Check sheet for the modelled part. Datum: model origin and axes. Units: mm. A direction names the side the tool comes from. Coordinates: 2 decimals unless noted, no trailing zeros. Loops run counter-clockwise (first coordinate to the right, second up) from the corner with the lowest first, then second, coordinate; pieces in that order, holes last. Notation, with made-up numbers: M -31.75,87 L 4.25,87 A18 ccw 4.25,92 Z; hole C -36.75,-27.75 d2. An arc over 180 degrees is marked long. Answer in a Markdown table with one row per item. Add a question column.
```python
from build123d import *

# Parameters (mm, degrees)
F0_W      = 50.8
F0_H      = 50.8
F1_DEPTH  = 4.13
F3_W      = 45.72
F3_H      = 45.72
F4_DEPTH  = 3.77
F5_W      = 8
F5_H      = 23.114
F6_DEPTH  = 3.2
F7_R      = 1.715
F8_DEPTH  = 25.4
F9_SIZE   = 1.27
F10_R     = 1.694213851
F11_DEPTH = 25.4


# Not quite as in the source:
# - a feature names something its author has since deleted; it is built from what else it names


with BuildPart() as f1:
    # F0 (on Top) → F1 (new body)
    with BuildSketch(Plane.XY):
        with Locations((13.0843408406, 14.7212249442)):
            Rectangle(F0_W, F0_H)
    extrude(amount=F1_DEPTH)

    # F3 (on face) → F4 (join)
    with BuildSketch(Plane.XY.offset(4.13)):
        with Locations((13.0843408406, 14.7212249442)):
            Rectangle(F3_W, F3_H)
    extrude(amount=F4_DEPTH)

    # F5 (on face) → F6 (cut)
    with BuildSketch(Plane.XY.offset(7.9)):
        with Locations((4.2001288666, 14.5942249442)):
            Rectangle(F5_W, F5_H)
        with Locations((13.0901288666, 14.5942249442)):
            Rectangle(F5_W, F5_H)
        with Locations((21.9801288666, 14.5942249442)):
            Rectangle(F5_W, F5_H)
        with Locations((30.8701288666, 14.5942249442)):
            Rectangle(F5_W, F5_H)
        with Locations((-4.6898711334, 14.5942249442)):
            Rectangle(F5_W, F5_H)
    extrude(amount=-F6_DEPTH, mode=Mode.SUBTRACT)

    # F7 (on face) → F8 (cut)
    with BuildSketch(Plane.XY.offset(4.7)):
        with Locations((-4.6898711334, 7.9362249442)):
            Circle(F7_R)
    extrude(amount=-F8_DEPTH, mode=Mode.SUBTRACT)

    # F9
    f9_edges = [f1.edges().sort_by_distance(p)[0] for p in [
        (13.084341, -10.678775, 0),
        (13.084341, 40.121225, 0),
        (-12.315659, 14.721225, 0),
        (38.484341, 14.721225, 0),
    ]]
    chamfer(f9_edges, length=F9_SIZE)

    # F10 (on face) → F11 (cut)
    with BuildSketch(Plane.XY.offset(4.7)):
        with Locations((4.1879288666, 7.9312249442)):
            Circle(F10_R)
        with Locations((13.0779288666, 7.9312249442)):
            Circle(F10_R)
        with Locations((21.9679288666, 7.9312249442)):
            Circle(F10_R)
        with Locations((30.8579288666, 7.9394249442)):
            Circle(F10_R)
    extrude(amount=-F11_DEPTH, mode=Mode.SUBTRACT)


solid = f1.part
```
Q1. Access from +Z, -Z, +X, -X, +Y, -Y to the whole of each face (thin tool, end or side, straight path). Record for faces 1 (the face through (20.275, 8.006, 2.383)), 2 (the face through (-9.776, 14, 6)), 3 (the face through (31, 15, 4.7)).
Q2. Cross-section at B-B (x = 22). Record the cut outline in (y, z).
Q3. Cross-section at D-D (x = 16.5). Record the cut outline in (y, z).
Q4. Thickness scan on L1, parallel to X at y = 14.5, z = 7.25; L2, parallel to Y at x = 18.5, z = 7; L3, parallel to Z at x = -8.5, y = 7. Record the ranges inside material, lowest first.
Q5. Cross-section at A-A (z = 6.75). Record the cut outline in (x, y), plus the area to 3 significant figures.
Q6. Go/stop test with flat-tipped pins: pin 1 (1 mm diameter, centred on x = 30, z = 6.5, fed in from +Y); pin 2 (1.5 mm diameter, centred on y = 22, z = 1, fed in from +X); pin 3 (1.6 mm diameter, centred on y = 18.5, z = 6.5, fed in from +X); pin 4 (1.9 mm diameter, centred on y = 13.5, z = 5.5, fed in from -X). Record where each tip stops, or that it passes through.
Q7. Mould release check, pull along X, two halves, no side actions. Record for faces 4 (the face through (13, -10.679, 3)), 5 (the face through (-12.316, 14, 3)), 6 (the face through (8.2, 14, 6)): released by +X, released by -X, zero draft, split by the parting line, or undercut.
Q8. Cross-section at C-C (y = 29). Record the cut outline in (x, z).
Answer key:
| question | item | result |
|---|---|---|
| 1 | face 1 | +Z, -Z |
| 1 | face 2 | +Z, -X, +Y, -Y |
| 1 | face 3 | +Z |
| 2 | outline | M -10.68,1.27 L -9.41,0 L 6.24,0 L 6.24,4.7 L 3.04,4.7 L 3.04,7.9 L -8.14,7.9 L -8.14,4.13 L -10.68,4.13 Z; M 9.63,0 L 38.85,0 L 40.12,1.27 L 40.12,4.13 L 37.58,4.13 L 37.58,7.9 L 26.15,7.9 L 26.15,4.7 L 9.63,4.7 Z |
| 3 | outline | M -10.68,1.27 L -9.41,0 L 38.85,0 L 40.12,1.27 L 40.12,4.13 L 37.58,4.13 L 37.58,7.9 L 26.15,7.9 L 26.15,4.7 L 3.04,4.7 L 3.04,7.9 L -8.14,7.9 L -8.14,4.13 L -10.68,4.13 Z |
| 4 | L1 | -9.78 to -8.69, -0.69 to 0.2, 8.2 to 9.09, 17.09 to 17.98, 25.98 to 26.87, 34.87 to 35.94 |
| 4 | L2 | -8.14 to 3.04, 26.15 to 37.58 |
| 4 | L3 | 0 to 4.7 |
| 5 | outline | M -9.78,-8.14 L 35.94,-8.14 L 35.94,37.58 L -9.78,37.58 Z; hole M -8.69,3.04 L -0.69,3.04 L -0.69,26.15 L -8.69,26.15 Z; hole M 0.2,3.04 L 8.2,3.04 L 8.2,26.15 L 0.2,26.15 Z; hole M 9.09,3.04 L 17.09,3.04 L 17.09,26.15 L 9.09,26.15 Z; hole M 17.98,3.04 L 25.98,3.04 L 25.98,26.15 L 17.98,26.15 Z; hole M 26.87,3.04 L 34.87,3.04 L 34.87,26.15 L 26.87,26.15 Z |
| 5 | area | 1,170 mm^2 |
| 6 | pin 1 | y = 37.58 |
| 6 | pin 2 | x = 38.48 |
| 6 | pin 3 | x = 35.94 |
| 6 | pin 4 | x = -9.78 |
| 7 | face 4 | zero draft |
| 7 | face 5 | released by -X |
| 7 | face 6 | undercut |
| 8 | outline | M -12.32,1.27 L -11.05,0 L 37.21,0 L 38.48,1.27 L 38.48,4.13 L 35.94,4.13 L 35.94,7.9 L -9.78,7.9 L -9.78,4.13 L -12.32,4.13 Z |
